Input: part model. Units: mm. Frame: model coordinates. Face numbers are marked on the shaded views. Round coordinates to 2 decimals unless told otherwise and drop trailing zeros. Loops run counter-clockwise (first coordinate to the right, second up) from the corner with the lowest first, then second, coordinate; pieces in that order, holes last. Notation, with made-up numbers: (77.25, 29.5) -> (132.25, 29.5) arc R21 cw to (132.25, 49.5) -> close; hole circle Ø9 at (73.5, 51.5). An arc over 180 degrees is marked (long way). Answer as a JSON object with one key per item and string values. Group by question number.
Item 1: Material intervals for line 1 (Z direction, x = -15, y = -32.5); line 2 (X direction, y = -36.5, z = 7); line 3 (X direction, y = -12, z = 5.5), sorted ascending. Write a range as [from, to].
Item 2: Pin query (flat end, axial travel): pin 1 (8.5 mm diameter, centred on x = 14.53, z = 8, fed in from -Y); pin 2 (6 mm diameter, centred on x = 20.5, z = 0, fed in from +Y); pin 3 (4 mm diameter, centred on x = -20.5, z = 16.5, fed in from +Y); pin 4 (4 mm diameter, centred on y = -9, z = -12.5, fed in from -X). Return the tip coordinate at first contact, or that it passes through.
Item 3: Section query A-A on z = -7. Return loops of the section in (x, y), and give its area (3 significant figures).
Item 4: Draft query along X for the marked faces 1, 2 and 3. Return one class per face: released by +X, released by -X, zero draft, split by the parting line, or undercut.
Item 5: Section query C-C on y = -10. Return loops of the section in (x, z), and give its area (3 significant figures).
Item 6: Section query B-B on x = 6.5. Return loops of the section in (y, z), and give its area (3 significant figures).
Item 7: Section query D-D on z = 6. Return loops of the section in (x, y), and give its area (3 significant figures).
from build123d import *

# Parameters (mm, degrees)
F0_W     = 59.375844
F0_H     = 45.479368
F1_DEPTH = 50.8
F2_SIZE  = 5.08
F3_R     = 12.7
F4_R     = 3.795792
F4_R_2   = 4.622578
F5_DEPTH = 50.8


with BuildPart() as f1:
    # F0 (on Front) → F1 (new body)
    with BuildSketch(Plane.XZ):
        Rectangle(F0_W, F0_H)
    extrude(amount=F1_DEPTH)

    # F2
    f2_edges = [f1.edges().sort_by_distance(p)[0] for p in [
        (0, -50.8, 22.739684),
        (29.687922, -50.8, 0),
        (0, -50.8, -22.739684),
        (-29.687922, -50.8, 0),
    ]]
    chamfer(f2_edges, length=F2_SIZE)

    # F3
    f3_edges = [f1.edges().sort_by_distance(p)[0] for p in [
        (29.687922, 0, 0),
        (0, 0, 22.739684),
        (-29.687922, 0, 0),
        (0, 0, -22.739684),
    ]]
    fillet(f3_edges, radius=F3_R)

    # F4 (on face) → F5 (cut)
    with BuildSketch(Plane.XZ.offset(50.8)):
        with Locations((-14.949238, 8.211552)):
            Circle(F4_R)
        with Locations((14.528131, 8.001001)):
            Circle(F4_R_2)
    extrude(amount=-F5_DEPTH, mode=Mode.SUBTRACT)


solid = f1.part
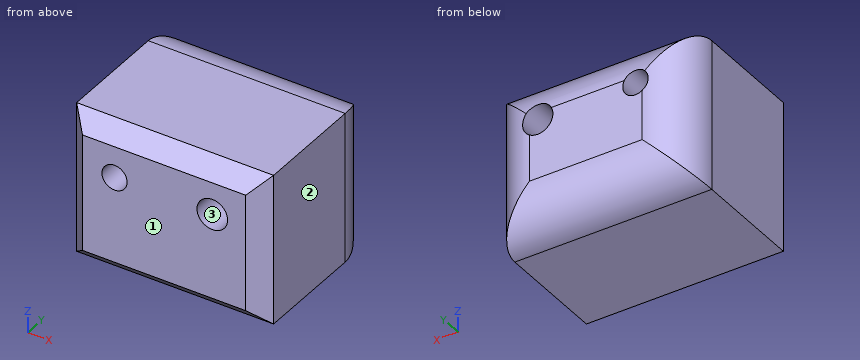
Solved:
{
 "1": {"line 1": "[-22.74, 4.42], [12.01, 22.74]", "line 2": "[-29.69, -18.55], [-11.35, 10.02], [19.04, 29.69]", "line 3": "[-29.67, -17.61], [-12.29, 10.64], [18.42, 29.67]"},
 "2": {"pin 1": "through", "pin 2": "y = -0.01", "pin 3": "y = -0.81", "pin 4": "x = -29.57"},
 "3": {"outline": "(-29.69, -45.72) -> (-24.61, -50.8) -> (24.61, -50.8) -> (29.69, -45.72) -> (29.69, -12.7) arc R12.7 ccw to (16.99, 0) -> (-16.99, 0) arc R12.7 ccw to (-29.69, -12.7) -> close", "area": "2,920 mm²"},
 "4": {"face 1": "zero draft", "face 2": "released by +X", "face 3": "undercut"},
 "5": {"outline": "(-29.4, -22.45) -> (29.4, -22.45) -> (29.4, 22.45) -> (-29.4, 22.45) -> close; hole circle Ø7.59 at (-14.95, 8.21); hole circle Ø9.25 at (14.53, 8)", "area": "2,530 mm²"},
 "6": {"outline": "(-50.8, -17.66) -> (-45.72, -22.74) -> (-12.7, -22.74) arc R12.7 ccw to (0, -10.04) -> (0, 10.04) arc R12.7 ccw to (-12.7, 22.74) -> (-45.72, 22.74) -> (-50.8, 17.66) -> close", "area": "2,220 mm²"},
 "7": {"outline": "(-29.69, -45.72) -> (-24.61, -50.8) -> (-18.03, -50.8) -> (-18.03, -0.04) arc R12.7 ccw to (-29.69, -12.7) -> close; (-11.86, -50.8) -> (10.36, -50.8) -> (10.36, 0) -> (-11.86, 0) -> close; (18.7, -50.8) -> (24.61, -50.8) -> (29.69, -45.72) -> (29.69, -12.7) arc R12.7 ccw to (18.7, -0.12) -> close", "area": "2,180 mm²"}
}
